Can you work these out from the model? Positions are in its coordinate system, mm. Round coordinates to 2 decimals unless told otherwise and drop trailing zeros. Loops run counter-clockwise (first coordinate to the right, second up) from the corner with the lowest first, then second, coordinate; pieces in that order, holes last. Notation, with made-up numbers: (-8, -16) -> (1, -16) arc R27 cw to (1, 8) -> close; hole circle Ø10 at (45, -17.75). An arc over 180 degrees is marked (long way). Write each question's results on one line, items separated by ' | '.
from build123d import *

# Parameters (mm, degrees)
SKETCH_W      = 45
SKETCH_H      = 45
PAD_DEPTH     = 0.1
THICKNESS_T   = 1.4
SKETCH001_W   = 44
SKETCH001_H   = 44
SKETCH001_W_2 = 42
SKETCH001_H_2 = 42
PAD001_DEPTH  = 1.8
SKETCH002_W   = 39
SKETCH002_H   = 39
PAD002_DEPTH  = 2.2


with BuildPart() as part:
    # Sketch → Pad (new body)
    with BuildSketch(Plane.XY):
        with Locations((22.5, 22.5)):
            Rectangle(SKETCH_W, SKETCH_H)
    extrude(amount=PAD_DEPTH)

    # Thickness
    thickness_openings = [part.faces().sort_by_distance(p)[0] for p in [
        (22.5, 22.5, 0.1),
    ]]
    offset(amount=THICKNESS_T, openings=thickness_openings)

    # Sketch001 → Pad001 (new body)
    with BuildSketch(Plane.XY):
        with Locations((22.5, 22.5)):
            Rectangle(SKETCH001_W, SKETCH001_H)
        with Locations((22.5, 22.5)):
            Rectangle(SKETCH001_W_2, SKETCH001_H_2, mode=Mode.SUBTRACT)
    extrude(amount=PAD001_DEPTH)

    # Sketch002 → Pad002 (new body)
    with BuildSketch(Plane.XY):
        with Locations((22.5, 22.5)):
            Rectangle(SKETCH002_W, SKETCH002_H)
    extrude(amount=PAD002_DEPTH)


solid = part.part
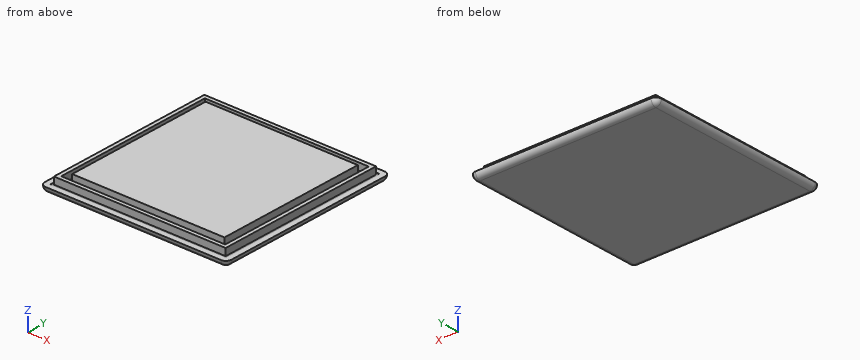
1. If we section it at A-A (z = 0.75): List the corners of the cut face in (x, y) for me, then the cut area to 3 significant figures.
Final values:
outline: (0.5, 0.5) -> (44.5, 0.5) -> (44.5, 44.5) -> (0.5, 44.5) -> close; (3, 3) -> (42, 3) -> (42, 42) -> (3, 42) -> close; hole (1.5, 1.5) -> (43.5, 1.5) -> (43.5, 43.5) -> (1.5, 43.5) -> close | area: 1,690 mm2
2. If we section it at B-B (y = 29): List the corners of the cut face in (x, z) for me.
Final values:
outline: (-1.4, 0) arc R1.4 ccw to (0, -1.4) -> (45, -1.4) arc R1.4 ccw to (46.4, 0) -> (46.4, 0.1) -> (45, 0.1) -> (45, 0) -> (44.5, 0) -> (44.5, 1.8) -> (43.5, 1.8) -> (43.5, 0) -> (42, 0) -> (42, 2.2) -> (3, 2.2) -> (3, 0) -> (1.5, 0) -> (1.5, 1.8) -> (0.5, 1.8) -> (0.5, 0) -> (0, 0) -> (0, 0.1) -> (-1.4, 0.1) -> close
3. Please list where these lines run through material, in increasing order: line 1 (Y direction, x = 32.5, z = 0.8); line 2 (X direction, y = 2, z = 1.15). Write a range as from..to.
Final values:
line 1: 0.5..1.5, 3..42, 43.5..44.5 | line 2: 0.5..1.5, 43.5..44.5
4. Will these pins go through, and if not, where does the flat tip stop? pin 1 (1 mm diameter, centred on x = 3.5, z = 1.5, fed in from +Y); pin 2 (2 mm diameter, centred on x = 18, z = 1, fed in from -Y); pin 3 (0.9 mm diameter, centred on y = 16.5, z = 1.5, fed in from -X); pin 4 (0.5 mm diameter, centred on x = 21, z = 0.5, fed in from -Y).
Final values:
pin 1: y = 44.5 | pin 2: y = -1.4 | pin 3: x = 0.5 | pin 4: y = 0.5
